```python
from build123d import *

# Parameters (mm, degrees)
BOSS_EXTRUDE1_DEPTH = 2.8
BOSS_EXTRUDE5_DEPTH = 2.8
BOSS_EXTRUDE2_DEPTH = 2.8
BOSS_EXTRUDE3_DEPTH = 2.8
BOSS_EXTRUDE4_DEPTH = 2.8
BOSS_EXTRUDE6_DEPTH = 11.2
BOSS_EXTRUDE7_START = -2.8
BOSS_EXTRUDE7_DEPTH = 2.8


with BuildPart() as part:
    # Sketch1 → Boss-Extrude1 (new body)
    with BuildSketch(Plane.XY):
        with BuildLine():
            Line((-31.75, 18.9), (31.75, 18.9))
            ThreePointArc((31.75, 18.9), (50.65, 0), (31.75, -18.9))
            Line((31.75, -18.9), (-31.75, -18.9))
            ThreePointArc((-31.75, -18.9), (-50.65, 0), (-31.75, 18.9))
        make_face()
    extrude(amount=BOSS_EXTRUDE1_DEPTH)

    # Sketch5 → Boss-Extrude5 (add)
    with BuildSketch(Plane(origin=(0, 0, 0), x_dir=(-1, 0, 0), z_dir=(0, 0, -1))):
        with BuildLine():
            Line((-46.65, -13.7), (-46.65, 13.7))
            ThreePointArc((-46.65, 13.7), (-37.937921505, 29.619053219), (-19.833465037, 30.862123242))
            Line((-19.833465037, 30.862123242), (9.866534963, 17.162123242))
            ThreePointArc((9.866534963, 17.162123242), (20.85, 0), (9.866534963, -17.162123242))
            Line((9.866534963, -17.162123242), (-19.833465037, -30.862123242))
            ThreePointArc((-19.833465037, -30.862123242), (-37.937921505, -29.619053219), (-46.65, -13.7))
        make_face()
    extrude(amount=BOSS_EXTRUDE5_DEPTH)

    # Sketch2 → Boss-Extrude2 (add)
    with BuildSketch(Plane.XY.offset(2.8)):
        with BuildLine():
            Line((-45.25, 18.9), (45.25, 18.9))
            ThreePointArc((45.25, 18.9), (64.15, 0), (45.25, -18.9))
            Line((45.25, -18.9), (-45.25, -18.9))
            ThreePointArc((-45.25, -18.9), (-64.15, 0), (-45.25, 18.9))
        make_face()
    extrude(amount=BOSS_EXTRUDE2_DEPTH)

    # Sketch3 → Boss-Extrude3 (add)
    with BuildSketch(Plane.XY.offset(5.6)):
        with BuildLine():
            Line((-58.75, 18.9), (58.75, 18.9))
            ThreePointArc((58.75, 18.9), (77.65, 0), (58.75, -18.9))
            Line((58.75, -18.9), (-58.75, -18.9))
            ThreePointArc((-58.75, -18.9), (-77.65, 0), (-58.75, 18.9))
        make_face()
    extrude(amount=BOSS_EXTRUDE3_DEPTH)

    # Sketch4 → Boss-Extrude4 (add)
    with BuildSketch(Plane.XY.offset(8.4)):
        with BuildLine():
            Line((-72.75, 18.9), (72.75, 18.9))
            ThreePointArc((72.75, 18.9), (91.65, 0), (72.75, -18.9))
            Line((72.75, -18.9), (-72.75, -18.9))
            ThreePointArc((-72.75, -18.9), (-91.65, 0), (-72.75, 18.9))
        make_face()
    extrude(amount=BOSS_EXTRUDE4_DEPTH)

    # Sketch7 → Boss-Extrude6 (add)
    with BuildSketch(Plane.XY):
        with BuildLine():
            Line((31.75, -18.9), (-6.099021116, -18.9))
            Line((-6.099021116, -18.9), (19.833465037, -30.862123242))
            ThreePointArc((19.833465037, -30.862123242), (37.937921505, -29.619053219), (46.65, -13.7))
            Line((46.65, -13.7), (46.65, -11.627553483))
            ThreePointArc((46.65, -11.627553483), (40.040031338, -16.984857386), (31.75, -18.9))
        make_face()
        with BuildLine():
            Line((46.65, 11.627553483), (46.65, 13.7))
            ThreePointArc((46.65, 13.7), (37.937921505, 29.619053219), (19.833465037, 30.862123242))
            Line((19.833465037, 30.862123242), (-6.099021116, 18.9))
            Line((-6.099021116, 18.9), (31.75, 18.9))
            ThreePointArc((31.75, 18.9), (40.040031338, 16.984857386), (46.65, 11.627553483))
        make_face()
    extrude(amount=BOSS_EXTRUDE6_DEPTH)

    # Sketch10 → Boss-Extrude7 (add)
    with BuildSketch(Plane(origin=(0, 0, -2.8), x_dir=(-1, 0, 0), z_dir=(0, 0, -1)).offset(BOSS_EXTRUDE7_START)):
        with BuildLine():
            ThreePointArc((18.009763314, -9.964637591), (28.85, 0), (18.009763314, 9.964637591))
            ThreePointArc((18.009763314, 9.964637591), (20.85, 0), (18.009763314, -9.964637591))
        make_face()
    extrude(amount=BOSS_EXTRUDE7_DEPTH)


solid = part.part
```
Check sheet for the modelled part. Datum: model origin and axes. Units: mm. A direction names the side the tool comes from. Coordinates: 2 decimals unless noted, no trailing zeros. Write each loop counter-clockwise with the first axis right and the second up, starting at its lowest first coordinate (ties: lowest second). Pieces come first, ordered by that corner, then holes. Notation, with made-up numbers: (-30, 11) -> (9, 11) arc R10 ccw to (9, 30) -> close; hole circle Ø6 at (76.5, 83.5). An arc over 180 degrees is marked (long way). Use a Markdown table: item, result.
1. Sectioned sample at A-A (y = 0). Enter the section's corners in (x, z).
Reported:
| item | result |
|---|---|
| outline | (-91.65, 8.4) -> (-77.65, 8.4) -> (-77.65, 5.6) -> (-64.15, 5.6) -> (-64.15, 2.8) -> (-50.65, 2.8) -> (-50.65, 0) -> (-28.85, 0) -> (-28.85, -2.8) -> (46.65, -2.8) -> (46.65, 0) -> (50.65, 0) -> (50.65, 2.8) -> (64.15, 2.8) -> (64.15, 5.6) -> (77.65, 5.6) -> (77.65, 8.4) -> (91.65, 8.4) -> (91.65, 11.2) -> (-91.65, 11.2) -> close |
2. Sectioned sample at D-D (x = 34.5). Enter the section's corners in (y, z).
Reported:
| item | result |
|---|---|
| outline | (-31.35, -2.8) -> (31.35, -2.8) -> (31.35, 11.2) -> (-31.35, 11.2) -> close |
3. Tool access check on faces 1 (the flat face through (57, -18.9, 9)), 2 (the flat face through (-32, 18.9, 7)), 3 (the cylindrical face through (-14.524, -14.11, -1.38)). Record the directions out of +Z, -Z, +X, -X, +Y, -Y that give a thin tool (end or side, any length) a straight path to the whole face; none if there is none.
Reported:
| item | result |
|---|---|
| face 1 | +Z, -Z, +X, -Y |
| face 2 | +Z, -Z, -X, +Y |
| face 3 | -Z, -X, -Y |
4. Sectioned sample at C-C (x = 6.5). Enter the section's corners in (y, z), plus the area to 3 significant figures.
Reported:
| item | result |
|---|---|
| outline | (-24.71, -2.8) -> (24.71, -2.8) -> (24.71, 11.2) -> (-24.71, 11.2) -> close |
| area | 692 mm2 |
5. Sectioned sample at B-B (x = -22). Enter the section's corners in (y, z), plus the area to 3 significant figures.
Reported:
| item | result |
|---|---|
| outline | (-18.9, 0) -> (-9.49, 0) -> (-9.49, -2.8) -> (9.49, -2.8) -> (9.49, 0) -> (18.9, 0) -> (18.9, 11.2) -> (-18.9, 11.2) -> close |
| area | 477 mm2 |
6. Go/stop test with flat-tipped pins: pin 1 Ø1 at (y, z) = (-7.5, 8) entering from +X; pin 2 Ø9.5 at (x, y) = (-54, 3.5) entering from -Z; pin 3 Ø8 at (y, z) = (-2, 3) entering from -X. Record where each tip stops, or that it passes through.
Reported:
| item | result |
|---|---|
| pin 1 | stops at x = 90.22 |
| pin 2 | stops at z = 0 |
| pin 3 | stops at x = -77.65 |
7. Scan lines: line 1 along Z through (x, y) = (56.5, 11.5); line 2 along Z through (x, y) = (-38.5, -1); line 3 along Y through (x, z) = (-24.5, 4.5). Record each from-to range of solid material in increasing order.
Reported:
| item | result |
|---|---|
| line 1 | z = 2.8 to 11.2 |
| line 2 | z = 0 to 11.2 |
| line 3 | y = -18.9 to 18.9 |
